Could you check a few things on this model? Use its own coordinates, in mm. Face numbers are marked on the shaded views. A direction names the side the tool comes from. Give positions to 0.01 mm unless a question says otherwise; leave off trailing zeros. Loops run counter-clockwise (first coordinate to the right, second up) from the corner with the lowest first, then second, coordinate; pieces in that order, holes last. Notation, with made-up numbers: (-7.75, 80.25) -> (21.25, 80.25) arc R8 cw to (21.25, 91.25) -> close; hole circle Ø3 at (10.5, 56). An arc over 180 degrees is marked (long way). Write item = value, one per line. Start each with the question number.
1) I want a section at B-B (x = 0). List the corners of the cut face in (y, z) for me, and give its area (3 significant figures).
2) I need wall thicknesses on probe 1 along Y at (x, z) = (0, 25); probe 2 along Y at (x, z) = (-16.5, 32); probe 3 along X at (y, z) = (1.5, 24). Which ranges of each line are inside material? Lowest first, please. Write a range as from..to.
3) I'm going to push a flat-ended pin straight in: pin 1 Ø0.5 at (x, y) = (2, 17) entering from +Z. Where does the tip first touch, or does it pass through?
4) I want a section at C-C (z = 32.5). List the corners of the cut face in (x, y) for me, and give its area (3 significant figures).
5) I want a section at A-A (y = 0). List the corners of the cut face in (x, z) for me, and give its area (3 significant figures).
6) I want a section at D-D (x = -11). List the corners of the cut face in (y, z) for me, and give its area (3 significant figures).
7) On a 3-axis mill with a long thin cutter (end or side, diameter ignored), from which of +Z, -Z, +X, -X, +Y, -Y can I reach the whole of each face in a straight line? I mean the marked faces 1, 2 and 3. Say none if no direction works.
from build123d import *

# Parameters (mm, degrees)
SKETCH_1_R      = 18
SKETCH_1_R_2    = 6
EXTRUDE_1_DEPTH = 5
SKETCH_2_W      = 42
SKETCH_2_H      = 35
SKETCH_2_R      = 6
EXTRUDE_2_DEPTH = 35.7


with BuildPart() as part:
    # 草图1 → 凸台-拉伸1 (new body)
    with BuildSketch(Plane.XY):
        Circle(SKETCH_1_R)
        Circle(SKETCH_1_R_2, mode=Mode.SUBTRACT)
    extrude(amount=EXTRUDE_1_DEPTH)

    # 草图2 → 凸台-拉伸2 (add)
    with BuildSketch(Plane.XY.offset(5)):
        with Locations((0, -1)):
            Rectangle(SKETCH_2_W, SKETCH_2_H)
        Circle(SKETCH_2_R, mode=Mode.SUBTRACT)
    extrude(amount=EXTRUDE_2_DEPTH)


solid = part.part
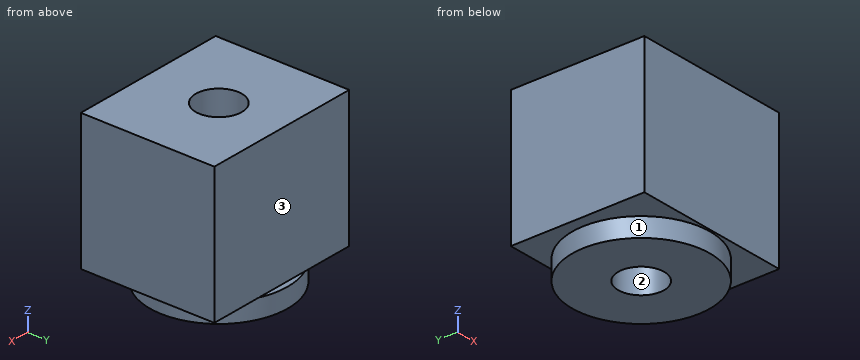
Answer list:
q1.outline = (-18.5, 5) -> (-18, 5) -> (-18, 0) -> (-6, 0) -> (-6, 40.7) -> (-18.5, 40.7) -> close; (6, 0) -> (18, 0) -> (18, 5) -> (16.5, 5) -> (16.5, 40.7) -> (6, 40.7) -> close
q1.area = 941 mm^2
q2.probe_1 = -18.5..-6, 6..16.5
q2.probe_2 = -18.5..16.5
q2.probe_3 = -21..-5.81, 5.81..21
q3.pin_1 = 5
q4.outline = (-21, -18.5) -> (21, -18.5) -> (21, 16.5) -> (-21, 16.5) -> close; hole circle Ø12 at (0, 0)
q4.area = 1,360 mm^2
q5.outline = (-21, 5) -> (-18, 5) -> (-18, 0) -> (-6, 0) -> (-6, 40.7) -> (-21, 40.7) -> close; (6, 0) -> (18, 0) -> (18, 5) -> (21, 5) -> (21, 40.7) -> (6, 40.7) -> close
q5.area = 1,190 mm^2
q6.outline = (-18.5, 5) -> (-14.25, 5) -> (-14.25, 0) -> (14.25, 0) -> (14.25, 5) -> (16.5, 5) -> (16.5, 40.7) -> (-18.5, 40.7) -> close
q6.area = 1,390 mm^2
q7.face_1 = -Z
q7.face_2 = +Z, -Z
q7.face_3 = +Z, +X, -X, +Y
